```python
from build123d import *

# Parameters (mm, degrees)
SKETCH1_W           = 41
SKETCH1_H           = 27
BOSS_EXTRUDE1_DEPTH = 10
SKETCH2_W           = 41
SKETCH2_H           = 5
BOSS_EXTRUDE2_DEPTH = 23
CUT_EXTRUDE1_REACH  = 35.638
SKETCH3_R           = 4


with BuildPart() as part:
    # Sketch1 → Boss-Extrude1 (new body)
    with BuildSketch(Plane.XY):
        Rectangle(SKETCH1_W, SKETCH1_H)
    extrude(amount=BOSS_EXTRUDE1_DEPTH)

    # Sketch2 → Boss-Extrude2 (add)
    with BuildSketch(Plane.XY.offset(10)):
        with Locations((0, 11)):
            Rectangle(SKETCH2_W, SKETCH2_H)
        with Locations((0, -11)):
            Rectangle(SKETCH2_W, SKETCH2_H)
    extrude(amount=BOSS_EXTRUDE2_DEPTH)

    # Sketch3 → Cut-Extrude1 (cut, up to next)
    with BuildSketch(Plane.XY.offset(10), mode=Mode.PRIVATE) as cut_extrude1_sk1:
        with Locations((-12.5, 0)):
            Circle(SKETCH3_R)
    cut_extrude1_tool1 = extrude(cut_extrude1_sk1.sketch, amount=-CUT_EXTRUDE1_REACH, mode=Mode.PRIVATE) & part.part
    # Sketch3 → Cut-Extrude1 (cut, up to next)
    with BuildSketch(Plane.XY.offset(10), mode=Mode.PRIVATE) as cut_extrude1_sk2:
        with Locations((12.5, 0)):
            Circle(SKETCH3_R)
    cut_extrude1_tool2 = extrude(cut_extrude1_sk2.sketch, amount=-CUT_EXTRUDE1_REACH, mode=Mode.PRIVATE) & part.part
    add(cut_extrude1_tool1.solids().sort_by_distance((-12.5, 0, 10))[0], mode=Mode.SUBTRACT)
    add(cut_extrude1_tool2.solids().sort_by_distance((12.5, 0, 10))[0], mode=Mode.SUBTRACT)


solid = part.part
```
Geometry check sheet. Reference: the model listing, model coordinates, mm. A direction names the side the tool comes from. Give positions to 0.01 mm unless a question says otherwise; leave off trailing zeros. Write each loop counter-clockwise with the first axis right and the second up, starting at its lowest first coordinate (ties: lowest second). Pieces come first, ordered by that corner, then holes.
1) Section check D-D, the plane z = 5.5. Record the boundary of the cut face in (x, y), and give its area (3 significant figures).
2) Section check C-C, the plane x = -12.5. Record the boundary of the cut face in (y, z).
3) Access from +Z, -Z, +X, -X, +Y, -Y to the whole of each face (thin tool, end or side, straight path). Record for faces 1 (the flat face through (-20.5, 0, 9)), 2 (the flat face through (0, 0, 10)).
4) Release check for a two-part mould opening along Y. For faces 3 (the flat face through (0, -8.5, 21)), 4 (the flat face through (20.5, 0, 9)), 5 (the flat face through (0, 13.5, 16)) record: pulls with the +Y half, pulls with the -Y half, needs draft (parallel to the pull), parting line crosses it, or undercut.
5) Section check A-A, the plane y = 0. Record the boundary of the cut face in (x, z), and give its area (3 significant figures).
6) Section check B-B, the plane z = 23.5. Record the boundary of the cut face in (x, y), and give its area (3 significant figures).
7) Gauge pin test, flat end, axial feed: pin 1 (1.5 mm diameter, centred on x = 9, y = 1, fed in from +Z). Record the tip position at first contact, or that the pin passes through.
8) Material ranges on L1, parallel to Y at x = -15.5, z = 27; L2, parallel to Y at x = 12.5, z = 5; L3, parallel to Z at x = -13.5, y = 4.5, recorded low to high.
Computed:
1. outline: (-20.5, -13.5) - (20.5, -13.5) - (20.5, 13.5) - (-20.5, 13.5) - close; hole circle Ø8 at (-12.5, 0); hole circle Ø8 at (12.5, 0)
1. area: 1,010 mm2
2. outline: (-13.5, 0) - (-4, 0) - (-4, 10) - (-8.5, 10) - (-8.5, 33) - (-13.5, 33) - close; (4, 0) - (13.5, 0) - (13.5, 33) - (8.5, 33) - (8.5, 10) - (4, 10) - close
3. face 1: +Z, -Z, -X, +Y, -Y
3. face 2: +Z, +X, -X
4. face 3: undercut
4. face 4: needs draft
4. face 5: pulls with the +Y half
5. outline: (-20.5, 0) - (-16.5, 0) - (-16.5, 10) - (-20.5, 10) - close; (-8.5, 0) - (8.5, 0) - (8.5, 10) - (-8.5, 10) - close; (16.5, 0) - (20.5, 0) - (20.5, 10) - (16.5, 10) - close
5. area: 250 mm2
6. outline: (-20.5, -13.5) - (20.5, -13.5) - (20.5, -8.5) - (-20.5, -8.5) - close; (-20.5, 8.5) - (20.5, 8.5) - (20.5, 13.5) - (-20.5, 13.5) - close
6. area: 410 mm2
7. pin 1: stops at z = 10
8. L1: y = -13.5 to -8.5, 8.5 to 13.5
8. L2: y = -13.5 to -4, 4 to 13.5
8. L3: z = 0 to 10
